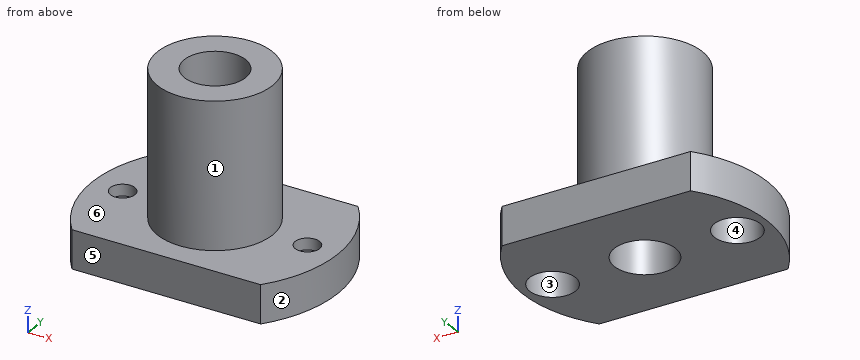
```python
from build123d import *

# Parameters (mm, degrees)
PAD_DEPTH       = 5
SKETCH001_R     = 1.6
POCKET_DEPTH    = 5.001
SKETCH002_R     = 7.5
PAD001_DEPTH    = 19
SKETCH003_R     = 4
POCKET001_DEPTH = 24.001
SKETCH004_R     = 3
POCKET002_DEPTH = 3.5


with BuildPart() as part:
    # Sketch → Pad (new body)
    with BuildSketch(Plane.XY):
        with BuildLine():
            Line((-12.25, -10.5), (12.25, -10.5))
            ThreePointArc((12.25, -10.5), (15.993585, 0), (12.25, 10.5))
            Line((12.25, 10.5), (-12.25, 10.5))
            ThreePointArc((-12.25, 10.5), (-16.007739, 0), (-12.25, -10.5))
        make_face()
    extrude(amount=PAD_DEPTH)

    # Sketch001 (on Face6 of Pad) → Pocket (cut, through all)
    with BuildSketch(Plane.XY.offset(5)):
        with Locations((-12, 0)):
            Circle(SKETCH001_R)
        with Locations((12, 0)):
            Circle(SKETCH001_R)
    extrude(amount=-POCKET_DEPTH, mode=Mode.SUBTRACT)

    # Sketch002 (on Face5 of Pocket) → Pad001 (join)
    with BuildSketch(Plane.XY.offset(5)):
        Circle(SKETCH002_R)
    extrude(amount=PAD001_DEPTH)

    # Sketch003 (on Face10 of Pad001) → Pocket001 (cut, through all)
    with BuildSketch(Plane.XY.offset(24)):
        Circle(SKETCH003_R)
    extrude(amount=-POCKET001_DEPTH, mode=Mode.SUBTRACT)

    # Sketch004 (on Face4 of Pocket001) → Pocket002 (cut)
    with BuildSketch(Plane(origin=(0, 0, 0), x_dir=(1, 0, 0), z_dir=(0, 0, -1))):
        with Locations((-12, 0)):
            Circle(SKETCH004_R)
        with Locations((12, 0)):
            Circle(SKETCH004_R)
    extrude(amount=-POCKET002_DEPTH, mode=Mode.SUBTRACT)


solid = part.part
```
CAD build for the part. Positions are in the model's coordinates, mm. Face numbers are marked on the shaded views. A direction names the side the tool comes from. Coordinates: 2 decimals unless noted, no trailing zeros. Write each loop counter-clockwise with the first axis right and the second up, starting at its lowest first coordinate (ties: lowest second). Pieces come first, ordered by that corner, then holes.
(1) Cut at D-D, the plane y = -5. List the corners of the cut face in (x, z), and give its area (3 significant figures).
(2) 3-axis set-ups, long thin cutter, end or side, ignore diameter. For the marked faces 4, 5 and 6: which of +Z, -Z, +X, -X, +Y, -Y reach the whole face in a straight line?
(3) Drill centre lines: probe 1 along Y at (x, z) = (12, 0.85); probe 2 along Y at (x, z) = (0, 12.5); probe 3 along Z at (x, y) = (9.5, 3). Where is each one in solid material? Low to high.
(4) Two-plate mould, pull along X, no slides. Class the marked faces 1, 2 and 3: +X half, -X half, draft (parallel to the pull), parting line (faces both ways), or undercut.
(5) Cut at C-C, the plane z = 17.25. List the corners of the cut face in (x, y), and give its area (3 significant figures).
(6) Cut at A-A, the plane y = 0. List the corners of the cut face in (x, z).
(7) Flat gauge pins, fed straight in: pin 1 (3 mm diameter, centred on x = 13, y = 0.5, fed in from -Z); pin 2 (3 mm diameter, centred on y = 1, z = 10, fed in from -X); pin 3 (5 mm diameter, centred on y = 3, z = 6, fed in from +X). Where does each tip first touch, or does it go through?
(8) Cut at B-B, the plane x = 0. List the corners of the cut face in (y, z), and give its area (3 significant figures).
Geometry says:
1. outline: (-15.23, 0) - (15.22, 0) - (15.22, 5) - (5.59, 5) - (5.59, 24) - (-5.59, 24) - (-5.59, 5) - (-15.23, 5) - close
1. area: 365 mm2
2. face 4: -Z
2. face 5: +Z, -Z, +X, -X, -Y
2. face 6: +Z
3. probe 1: y = -10.5 to -3, 3 to 10.5
3. probe 2: y = -7.5 to -4, 4 to 7.5
3. probe 3: z = 0 to 5
4. face 1: parting line
4. face 2: +X half
4. face 3: undercut
5. outline: circle Ø15 at (0, 0); hole circle Ø8 at (0, 0)
5. area: 126 mm2
6. outline: (-16.01, 0) - (-15, 0) - (-15, 3.5) - (-13.6, 3.5) - (-13.6, 5) - (-16.01, 5) - close; (-10.4, 3.5) - (-9, 3.5) - (-9, 0) - (-4, 0) - (-4, 24) - (-7.5, 24) - (-7.5, 5) - (-10.4, 5) - close; (4, 0) - (9, 0) - (9, 3.5) - (10.4, 3.5) - (10.4, 5) - (7.5, 5) - (7.5, 24) - (4, 24) - close; (13.6, 3.5) - (15, 3.5) - (15, 0) - (15.99, 0) - (15.99, 5) - (13.6, 5) - close
7. pin 1: stops at z = 3.5
7. pin 2: stops at x = -7.5
7. pin 3: stops at x = 15.98
8. outline: (-10.5, 0) - (-4, 0) - (-4, 24) - (-7.5, 24) - (-7.5, 5) - (-10.5, 5) - close; (4, 0) - (10.5, 0) - (10.5, 5) - (7.5, 5) - (7.5, 24) - (4, 24) - close
8. area: 198 mm2
